Geometry check sheet. Reference: the model listing, model coordinates, mm. Face numbers are marked on the shaded views. A direction names the side the tool comes from. Coordinates: 2 decimals unless noted, no trailing zeros. Write each loop counter-clockwise with the first axis right and the second up, starting at its lowest first coordinate (ties: lowest second). Pieces come first, ordered by that corner, then holes. Notation, with made-up numbers: (-22.75, -5.75) -> (-10.75, -5.75) arc R26 cw to (-10.75, 12.25) -> close; hole circle Ø6 at (40, 37). An arc over 180 degrees is marked (long way). One line per question, with ' | ' between items.
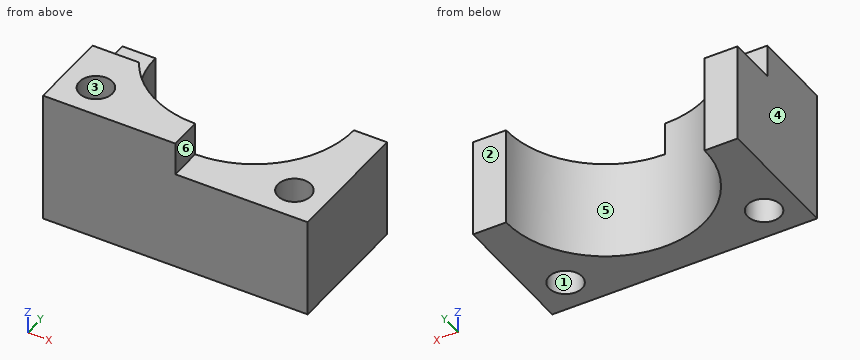
```python
from build123d import *

# Parameters (mm, degrees)
F0_R     = 5
F1_DEPTH = 40
F2_R     = 5
F3_DEPTH = 10


with BuildPart() as f1:
    # F0 (on Top) → F1 (new body)
    with BuildSketch(Plane.XY):
        with BuildLine():
            ThreePointArc((30, 0), (0, -30), (-30, 0))
            Line((-30, 0), (-40, 0))
            Line((-40, 0), (-40, -40))
            Line((-40, -40), (40, -40))
            Line((40, -40), (40, 0))
            Line((40, 0), (30, 0))
        make_face()
        with Locations((-30, -30)):
            Circle(F0_R, mode=Mode.SUBTRACT)
        with Locations((30, -30)):
            Circle(F0_R, mode=Mode.SUBTRACT)
    extrude(amount=F1_DEPTH)

    # F2 (on face) → F3 (cut)
    with BuildSketch(Plane.XY.offset(40)):
        with BuildLine():
            Line((-40, 0), (-40, -15))
            Line((-40, -15), (-25.980762, -15))
            ThreePointArc((-25.980762, -15), (-28.977775, -7.764571), (-30, 0))
            Line((-30, 0), (-40, 0))
        make_face()
        with BuildLine():
            ThreePointArc((30, 0), (21.213203, -21.213203), (0, -30))
            Line((0, -30), (0, -40))
            Line((0, -40), (40, -40))
            Line((40, -40), (40, 0))
            Line((40, 0), (30, 0))
        make_face()
        with Locations((30, -30)):
            Circle(F2_R, mode=Mode.SUBTRACT)
    extrude(amount=-F3_DEPTH, mode=Mode.SUBTRACT)


solid = f1.part
```
(1) Cross-section at D-D (y = -29). Record the cut outline in (x, z).
Answers below:
outline: (-40, 0) -> (-34.9, 0) -> (-34.9, 40) -> (-40, 40) -> close; (-25.1, 0) -> (-7.68, 0) -> (-7.68, 40) -> (-25.1, 40) -> close; (7.68, 0) -> (25.1, 0) -> (25.1, 30) -> (7.68, 30) -> close; (34.9, 0) -> (40, 0) -> (40, 30) -> (34.9, 30) -> close
(2) Cross-section at C-C (x = 29). Record the cut outline in (y, z), plus the area to 3 significant figures.
Answers below:
outline: (-40, 0) -> (-34.9, 0) -> (-34.9, 30) -> (-40, 30) -> close; (-25.1, 0) -> (-7.68, 0) -> (-7.68, 30) -> (-25.1, 30) -> close | area: 676 mm²
(3) Cross-section at B-B (z = 14). Record the cut outline in (x, y), plus the area to 3 significant figures.
Answers below:
outline: (-40, -40) -> (40, -40) -> (40, 0) -> (30, 0) arc R30 cw to (-30, 0) -> (-40, 0) -> close; hole circle Ø10 at (-30, -30); hole circle Ø10 at (30, -30) | area: 1,630 mm²
(4) Material ranges on line 1 (X direction, y = -34, z = 10.5); line 2 (Z direction, x = 21, y = -31.5); line 3 (Y direction, x = 1, z = 3), recorded low to high.
Answers below:
line 1: x = -40 to -33, -27 to 27, 33 to 40 | line 2: z = 0 to 30 | line 3: y = -40 to -29.98
(5) Cross-section at A-A (y = -20). Record the cut outline in (x, z), plus the area to 3 significant figures.
Answers below:
outline: (-40, 0) -> (-22.36, 0) -> (-22.36, 40) -> (-40, 40) -> close; (22.36, 0) -> (40, 0) -> (40, 30) -> (22.36, 30) -> close | area: 1,230 mm²
(6) Depth check by flat-ended pin: P1, Ø1.5, axis at y = -7, z = 31, coming from the +X side; P2, Ø2, axis at x = -21, z = 6.5, coming from the +Y side; P3, Ø3, axis at y = -36.5, z = 35.5, coming from the +X side; P4, Ø5, axis at x = -36, z = 36.5, coming from the +Y side. Enter the tip coordinate at first touch or a pass-through.
Answers below:
P1: passes through | P2: stops at y = -20.4 | P3: stops at x = 0 | P4: stops at y = -15
(7) Tool access check on the marked faces 5 and 6. Record the directions out of +Z, -Z, +X, -X, +Y, -Y that give a thin tool (end or side, any length) a straight path to the whole face; none if there is none.
Answers below:
face 5: +Z, -Z, +Y | face 6: +Z, +X, +Y, -Y
(8) Draft check along Y on the marked faces 1, 2, 3 and 4. Enter one of: pulls with the +Y half, pulls with the -Y half, needs draft (parallel to the pull), parting line crosses it, or undercut.
Answers below:
face 1: undercut | face 2: pulls with the +Y half | face 3: undercut | face 4: needs draft
